Read the model definition and answer for the solid it produces. Units are mm, in the model's axes. A direction names the side the tool comes from. Give positions to 0.01 mm unless a question says otherwise; leave off trailing zeros. Order: outer loops, then holes, each group sorted by start corner. A loop starts at its lowest first (then second) coordinate and runs counter-clockwise, first axis right, second up. Notation, with made-up numbers: (-8.75, -29.5) -> (50.25, -29.5) arc R15 cw to (50.25, -17.5) -> close; hole circle Ø7 at (34, 47.5). An arc over 180 degrees is marked (long way). One line per question, with ' | ' between items. Start each with the question number.
```python
from build123d import *

# Parameters (mm, degrees)
F0_R         = 11
F1_DEPTH     = 25.4
F2_W         = 4.2610359378
F2_H         = 5.4936911911
F1_FACE1_R   = 11
F3_DEPTH     = 25.401
F6_SIZE      = 4
F7_T1_DEPTH  = 5.4936911911
F7_T3_DEPTH  = 4.2610359378
F7_T11_DEPTH = 15.7804231429
F7_S13_R     = 11
F7_T14_DEPTH = 10
F7_T17_DEPTH = 14.5477678897
F7_S19_R     = 11
F7_T20_DEPTH = 9
F7_T26_DEPTH = 15.7804231429
F7_T30_DEPTH = 14.5477678897
F7_T37_DEPTH = 14.5477678897
F7_S39_R     = 11
F7_T40_DEPTH = 9
F7_T43_DEPTH = 15.7804231429
F7_S45_R     = 11
F7_T46_DEPTH = 10
F7_T52_DEPTH = 15.7804231429
F7_S54_R     = 11
F7_T55_DEPTH = 10
F7_T58_DEPTH = 14.5477678897
F7_S60_R     = 11
F7_T61_DEPTH = 9


# Not quite as in the source:
# - a fillet or chamfer that OpenCascade refuses, or shapes differently, is made with other operations: its cross-section is extruded or revolved along the edge and cut away or added


with BuildPart() as f1:
    # F0 (on Top) → F1 (new body)
    with BuildSketch(Plane.XY):
        Circle(F0_R)
    extrude(amount=F1_DEPTH)

    # F2 (on face) + F1_face1 (on face) → F3 (cut, through all)
    with BuildSketch(Plane.XY.offset(25.4)):
        with Locations((2.1305179689, 2.7468455955)):
            Rectangle(F2_W, F2_H)
    with BuildSketch(Plane(origin=(0, 0, 0), x_dir=(1, 0, 0), z_dir=(0, 0, -1))):
        Circle(F1_FACE1_R)
    extrude(amount=-F3_DEPTH, dir=(0, 0, 1), mode=Mode.SUBTRACT)

    # F4: fillet of radius 5.08 on 1 edges, made by hand

    # F4_s1 → F4_t2 (revolve, cut)
    with BuildSketch(Plane.XZ):
        with BuildLine():
            ThreePointArc((11, 5.08), (9.5121024484, 1.4878975516), (5.92, 0))
            Line((5.92, 0), (11, 0))
            Line((11, 0), (11, 5.08))
        make_face()
    revolve(axis=Axis((0, 0, 0), (0, 0, 1)), mode=Mode.SUBTRACT)

    # F5: F1 across face


with BuildPart() as f1_1:
    add(f1.part)
    add(f1.part.mirror(Plane(origin=(-0.5175939516, -0.6620763979, 0), x_dir=(1, 0, 0), z_dir=(0, 0, -1))))

    # F6
    f6_edges = [f1_1.edges().sort_by_distance(p)[0] for p in [
        (-11, 0, -25.4),
    ]]
    chamfer(f6_edges, length=F6_SIZE)

    # F7: chamfer of 4 on 5 edges, made by hand

    # F7_s2 → F7_t1 (cut)
    with BuildSketch(Plane.XZ.offset(-5.4936911911)):
        Polygon((0, 21.4), (-4, 25.4), (0, 25.4), align=None)
        Polygon((4.2610359378, 21.4), (8.2610359378, 25.4), (4.2610359378, 25.4), align=None)
    extrude(amount=F7_T1_DEPTH, mode=Mode.SUBTRACT)

    # F7_s4 → F7_t3 (cut)
    with BuildSketch(Plane.YZ):
        Polygon((0, 21.4), (-4, 25.4), (0, 25.4), align=None)
        Polygon((5.4936911911, 21.4), (9.4936911911, 25.4), (5.4936911911, 25.4), align=None)
    extrude(amount=F7_T3_DEPTH, mode=Mode.SUBTRACT)

    # F7_s5 → F7_t6 (revolve, cut)
    with BuildSketch(Plane.XZ):
        Polygon((7, 25.4), (11, 21.4), (11, 25.4), align=None)
    revolve(axis=Axis((0, 0, 25.4), (0, 0, 1)), mode=Mode.SUBTRACT)


with BuildPart() as f7_tool9:
    # F7_s10 → F7_t11 (new body)
    with BuildSketch(Plane.XZ.offset(-15.7804231429)):
        Polygon((0, 21.4), (-4, 25.4), (0, 25.4), align=None)
    extrude(amount=F7_T11_DEPTH)

    split(bisect_by=Plane.XZ.offset(-5.4936911911), keep=Keep.BOTTOM)

    # F7_s13 → F7_t14 (intersect, symmetric)
    with BuildSketch(Plane.XY.offset(23.4)):
        Circle(F7_S13_R)
    extrude(amount=F7_T14_DEPTH, both=True, mode=Mode.INTERSECT)


with BuildPart() as f7_tool15:
    # F7_s16 → F7_t17 (new body)
    with BuildSketch(Plane.YZ.offset(4.2610359378)):
        Polygon((5.4936911911, 21.4), (9.4936911911, 25.4), (5.4936911911, 25.4), align=None)
    extrude(amount=-F7_T17_DEPTH)

    split(bisect_by=Plane.YZ, keep=Keep.BOTTOM)

    # F7_s19 → F7_t20 (intersect, symmetric)
    with BuildSketch(Plane.XY.offset(23.4)):
        Circle(F7_S19_R)
    extrude(amount=F7_T20_DEPTH, both=True, mode=Mode.INTERSECT)


with BuildPart() as f7_tool9_1:
    add(f7_tool9.part)

    # F7_t21: intersect F7_tool15
    add(f7_tool15.part, mode=Mode.INTERSECT)


with BuildPart() as f1_2:
    add(f1_1.part)

    # F7_t7: cut F7_tool9
    add(f7_tool9_1.part, mode=Mode.SUBTRACT)


with BuildPart() as f7_tool24:
    # F7_s25 → F7_t26 (new body)
    with BuildSketch(Plane.XZ.offset(-5.4936911911)):
        Polygon((0, 21.4), (-4, 25.4), (0, 25.4), align=None)
    extrude(amount=F7_T26_DEPTH)

    split(bisect_by=Plane.XZ, keep=Keep.TOP)


with BuildPart() as f7_tool28:
    # F7_s29 → F7_t30 (new body)
    with BuildSketch(Plane.YZ.offset(-10.2867319519)):
        Polygon((0, 21.4), (-4, 25.4), (0, 25.4), align=None)
    extrude(amount=F7_T30_DEPTH)

    split(bisect_by=Plane.YZ, keep=Keep.BOTTOM)


with BuildPart() as f7_tool24_1:
    add(f7_tool24.part)

    # F7_t32: intersect F7_tool28
    add(f7_tool28.part, mode=Mode.INTERSECT)


with BuildPart() as f1_3:
    add(f1_2.part)

    # F7_t22: cut F7_tool24
    add(f7_tool24_1.part, mode=Mode.SUBTRACT)


with BuildPart() as f7_tool35:
    # F7_s36 → F7_t37 (new body)
    with BuildSketch(Plane.YZ):
        Polygon((0, 21.4), (-4, 25.4), (0, 25.4), align=None)
    extrude(amount=F7_T37_DEPTH)

    split(bisect_by=Plane.YZ.offset(4.2610359378), keep=Keep.TOP)

    # F7_s39 → F7_t40 (intersect, symmetric)
    with BuildSketch(Plane.XY.offset(23.4)):
        Circle(F7_S39_R)
    extrude(amount=F7_T40_DEPTH, both=True, mode=Mode.INTERSECT)


with BuildPart() as f7_tool41:
    # F7_s42 → F7_t43 (new body)
    with BuildSketch(Plane.XZ.offset(10.2867319519)):
        Polygon((4.2610359378, 21.4), (8.2610359378, 25.4), (4.2610359378, 25.4), align=None)
    extrude(amount=-F7_T43_DEPTH)

    split(bisect_by=Plane.XZ, keep=Keep.TOP)

    # F7_s45 → F7_t46 (intersect, symmetric)
    with BuildSketch(Plane.XY.offset(23.4)):
        Circle(F7_S45_R)
    extrude(amount=F7_T46_DEPTH, both=True, mode=Mode.INTERSECT)


with BuildPart() as f7_tool35_1:
    add(f7_tool35.part)

    # F7_t47: intersect F7_tool41
    add(f7_tool41.part, mode=Mode.INTERSECT)


with BuildPart() as f1_4:
    add(f1_3.part)

    # F7_t33: cut F7_tool35
    add(f7_tool35_1.part, mode=Mode.SUBTRACT)


with BuildPart() as f7_tool50:
    # F7_s51 → F7_t52 (new body)
    with BuildSketch(Plane.XZ):
        Polygon((4.2610359378, 21.4), (8.2610359378, 25.4), (4.2610359378, 25.4), align=None)
    extrude(amount=-F7_T52_DEPTH)

    split(bisect_by=Plane.XZ.offset(-5.4936911911), keep=Keep.BOTTOM)

    # F7_s54 → F7_t55 (intersect, symmetric)
    with BuildSketch(Plane.XY.offset(23.4)):
        Circle(F7_S54_R)
    extrude(amount=F7_T55_DEPTH, both=True, mode=Mode.INTERSECT)


with BuildPart() as f7_tool56:
    # F7_s57 → F7_t58 (new body)
    with BuildSketch(Plane.YZ.offset(14.5477678897)):
        Polygon((5.4936911911, 21.4), (9.4936911911, 25.4), (5.4936911911, 25.4), align=None)
    extrude(amount=-F7_T58_DEPTH)

    split(bisect_by=Plane.YZ.offset(4.2610359378), keep=Keep.TOP)

    # F7_s60 → F7_t61 (intersect, symmetric)
    with BuildSketch(Plane.XY.offset(23.4)):
        Circle(F7_S60_R)
    extrude(amount=F7_T61_DEPTH, both=True, mode=Mode.INTERSECT)


with BuildPart() as f7_tool50_1:
    add(f7_tool50.part)

    # F7_t62: intersect F7_tool56
    add(f7_tool56.part, mode=Mode.INTERSECT)


with BuildPart() as f1_5:
    add(f1_4.part)

    # F7_t48: cut F7_tool50
    add(f7_tool50_1.part, mode=Mode.SUBTRACT)


solid = f1_5.part
```
Q1. Determine the mould class of faces 1 (the flat face through (5.92, 2.13, 23.06)), 2 (the conical face through (-5.754, -4.412, 25.15)), 3 (the flat face through (-2.1, -4.4, 25.4)) for opening direction X: pulls with the +X half, pulls with the -X half, needs draft (parallel to the pull), parting line crosses it, or undercut.
Q2. Find the intervals of material crossed by line 1 (Z direction, x = 9, y = 5); line 2 (Z direction, x = 2, y = -10); line 3 (X direction, y = 4.5, z = 18), in increasing order.
Q3. Given P1, Ø1, axis at x = 7, z = -19, coming from the -Y side; P2, Ø5, axis at x = 9, z = -18, coming from the +Y side; P3, Ø1.6, axis at y = 1.5, z = 0.5, coming from the -X side, each flat-ended and moving along its own axis, determine where each tip first touches the part or whether it passes through.
Q4. Which of the six approach directions +Z, -Z, +X, -X, +Y, -Y give full straight-line access (tool end or side, diameter ignored) to faces 4 (the conical face through (-1.56, -7.02, -25.21)), 5 (the flat face through (-2, 2.1, 23.4)), 6 (the flat face through (2, 5.494, -2))?
Q5. A cutting plane is placed at A-A, the plane z = 16.5. Determine the outline of the cut face in (x, y), then the cut area to 3 significant figures.
Geometry results:
1) face 1: undercut | face 2: parting line crosses it | face 3: needs draft
2) line 1: -22.1 to -2.5, 2.5 to 22.1 | line 2: -22.2 to -2.34, 2.34 to 22.2 | line 3: -10.04 to 0, 4.26 to 10.04
3) P1: y = -8.87 | P2: y = 8.87 | P3: x = -9.2
4) face 4: -Z | face 5: +Z | face 6: +Z, -Z
5) outline: circle Ø22 at (0, 0); hole (0, 0) -> (4.26, 0) -> (4.26, 5.49) -> (0, 5.49) -> close | area: 357 mm²
